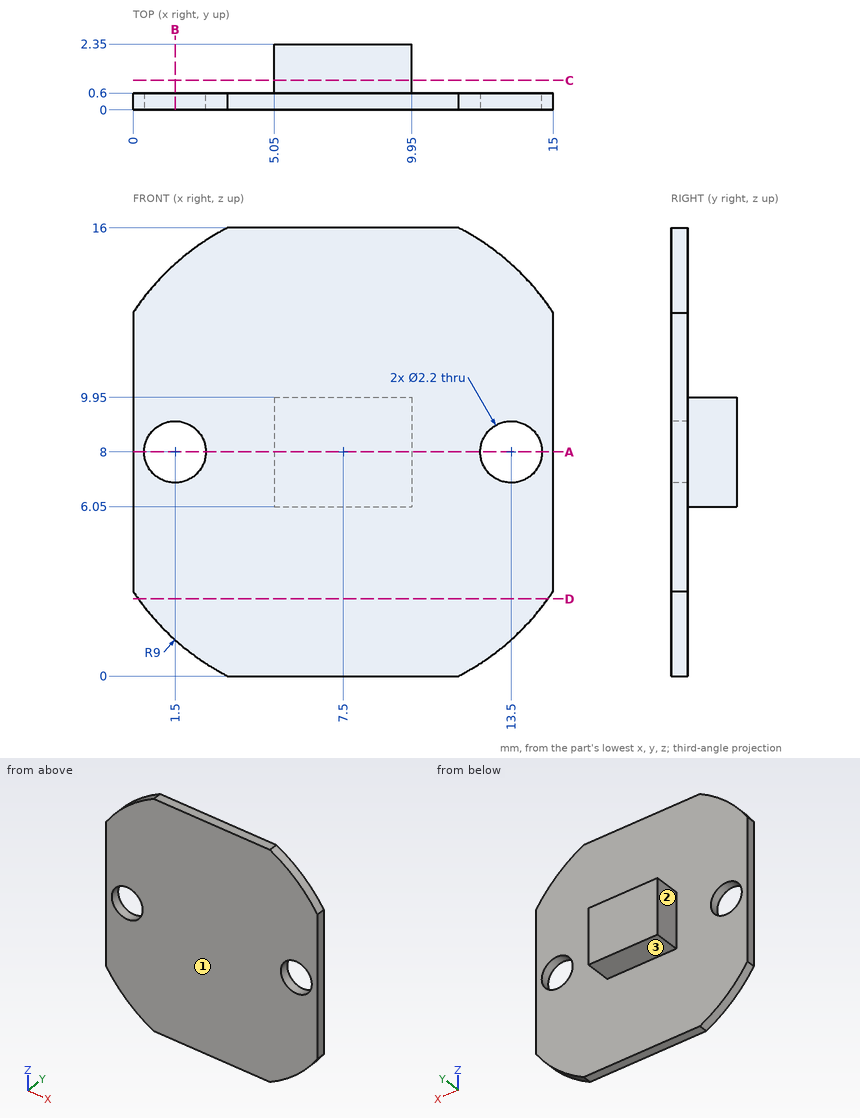
Check sheet for the drawn part. Datum: minimum x, y, z corner. Units: mm. A direction names the side the tool comes from. Give positions to 0.01 mm unless a question says otherwise; leave off trailing zeros. Order: outer loops, then holes, each group sorted by start corner. A loop starts at its lowest first (then second) coordinate and runs counter-clockwise, first axis right, second up. Notation, with made-up numbers: (16, -11) - (50, -11) arc R33 cw to (50, 26) - close; hole circle Ø4 at (26, 80). An arc over 180 degrees is marked (long way). Answer as a JSON object with one key per item and string values.
(1) Material ranges on line 1 (Y direction, x = 4.5, z = 7.75); line 2 (Z direction, x = 1.5, y = 0.3); line 3 (X direction, y = 1.25, z = 7.25), recorded low to high.
Report:
{"line 1": "0 to 0.6", "line 2": "1.29 to 6.9, 9.1 to 14.71", "line 3": "5.05 to 9.95"}
(2) Cross-section at B-B (x = 1.5). Record the cut outline in (y, z), then the cut area to 3 significant figures.
Report:
{"outline": "(0, 1.29) - (0.6, 1.29) - (0.6, 6.9) - (0, 6.9) - close; (0, 9.1) - (0.6, 9.1) - (0.6, 14.71) - (0, 14.71) - close", "area": "6.73 mm^2"}
(3) Cross-section at A-A (z = 8). Record the cut outline in (x, y), then the cut area to 3 significant figures.
Report:
{"outline": "(0, 0) - (0.4, 0) - (0.4, 0.6) - (0, 0.6) - close; (2.6, 0) - (12.4, 0) - (12.4, 0.6) - (9.95, 0.6) - (9.95, 2.35) - (5.05, 2.35) - (5.05, 0.6) - (2.6, 0.6) - close; (14.6, 0) - (15, 0) - (15, 0.6) - (14.6, 0.6) - close", "area": "14.9 mm^2"}
(4) Tool access check on the marked faces 1, 2 and 3. Record the directions out of +Z, -Z, +X, -X, +Y, -Y that give a thin tool (end or side, any length) a straight path to the whole face; none if there is none.
Report:
{"face 1": "+Z, -Z, +X, -X, -Y", "face 2": "+Z, -Z, -X, +Y", "face 3": "-Z, +X, -X, +Y"}
(5) Depth check by flat-ended pin: pin 1 Ø0.5 at (x, y) = (7.5, 1) entering from -Z; pin 2 Ø1.3 at (x, z) = (1.5, 8) entering from -Y; pin 3 Ø8 at (x, z) = (11, 14) entering from +Y. Enter the tip coordinate at first touch or a pass-through.
Report:
{"pin 1": "z = 6.05", "pin 2": "through", "pin 3": "y = 0.6"}
(6) Cross-section at C-C (y = 1.05). Record the cut outline in (x, z), then the cut area to 3 significant figures.
Report:
{"outline": "(5.05, 6.05) - (9.95, 6.05) - (9.95, 9.95) - (5.05, 9.95) - close", "area": "19.1 mm^2"}
(7) Cross-section at D-D (z = 2.75). Record the cut outline in (x, y).
Report:
{"outline": "(0.19, 0) - (14.81, 0) - (14.81, 0.6) - (0.19, 0.6) - close"}
